Check sheet for the modelled part. Datum: model origin and axes. Units: mm. A direction names the side the tool comes from. Round coordinates to 2 decimals unless told otherwise and drop trailing zeros. Write each loop counter-clockwise with the first axis right and the second up, starting at its lowest first coordinate (ties: lowest second). Pieces come first, ordered by that corner, then holes. Notation, with made-up numbers: (71.5, 24) - (116.5, 24) arc R4 cw to (116.5, 28) - close; hole circle Ø3 at (-5, 74). An arc over 180 degrees is marked (long way). Answer as a JSON object with one key per item and string values. Group by question number.
Item 1: Sectioned sample at C-C on x = 1.25. Record the boundary of the cut face in (y, z), plus the area to 3 significant figures.
Item 2: Sectioned sample at B-B on y = 2.5. Record the boundary of the cut face in (x, z).
Item 3: Sectioned sample at A-A on x = 6.25. Record the boundary of the cut face in (y, z).
Item 4: Gauge pin test, flat ends, axial feed: P1, Ø2.5, axis at y = 0, z = 7, coming from the +X side; P2, Ø1.5, axis at x = 1.5, z = 5, coming from the -Y side; P3, Ø8, axis at y = 6, z = 13.5, coming from the +X side. Record the tip position at first contact, or that the pin passes through.
Item 5: Release check for a two-part mould opening along Y. For faces 1 (the flat face through (5.458, -4.067, 9.86)), 2 (the flat face through (-2.75, 0, 10)), 3 (the flat face through (0.1, 3.4, 0)) record: pulls with the +Y half, pulls with the -Y half, needs draft (parallel to the pull), parting line crosses it, or undercut.
Item 6: Thickness scan on line 1 (X direction, y = 1, z = 13.5); line 2 (Y direction, x = 2.5, z = 10.5); line 3 (X direction, y = 2.5, z = 11.25). Record the ranges inside material, lowest first.
Item 7: Set-up check for faces 4 (the flat face through (-2.69, 6.25, 9.86)), 5 (the flat face through (-6.74, -0.815, 9.86)), 6 (the flat face through (-1.394, -2.37, 9.86)): record each of +Z, -Z, +X, -X, +Y, -Y from which the full face is reachable in a straight line by a thin tool's end or side.
```python
from build123d import *

# Parameters (mm, degrees)
PAD_DEPTH = 20


with BuildPart() as part:
    # Sketch → Pad (new body)
    with BuildSketch(Plane.XY):
        Polygon((-3.75, 6.495191), (-1.607695, 6), (0, 7.5), (1.607695, 6), (3.75, 6.495191), (4.392305, 4.392305), (6.495191, 3.75), (6, 1.607695), (7.5, 0), (6, -1.607695), (6.495191, -3.75), (4.392305, -4.392305), (3.75, -6.495191), (1.607695, -6), (0, -7.5), (-1.607695, -6), (-3.75, -6.495191), (-4.392305, -4.392305), (-6.495191, -3.75), (-6, -1.607695), (-7.5, 0), (-6, 1.607695), (-6.495191, 3.75), (-4.392305, 4.392305), align=None)
        Polygon((2.75, 1.587713), (0, 3.175426), (-2.75, 1.587713), (-2.75, -1.587713), (0, -3.175426), (2.75, -1.587713), align=None, mode=Mode.SUBTRACT)
    extrude(amount=PAD_DEPTH)


solid = part.part
```
Completed:
{
 "1": {"outline": "(-6.33, 0) - (-2.45, 0) - (-2.45, 20) - (-6.33, 20) - close; (2.45, 0) - (6.33, 0) - (6.33, 20) - (2.45, 20) - close", "area": "155 mm²"},
 "2": {"outline": "(-6.21, 0) - (-1.17, 0) - (-1.17, 20) - (-6.21, 20) - close; (1.17, 0) - (6.21, 0) - (6.21, 20) - (1.17, 20) - close"},
 "3": {"outline": "(-3.82, 0) - (-2.69, 0) - (-2.69, 20) - (-3.82, 20) - close; (-1.34, 0) - (1.34, 0) - (1.34, 20) - (-1.34, 20) - close; (2.69, 0) - (3.82, 0) - (3.82, 20) - (2.69, 20) - close"},
 "4": {"P1": "x = 7.5", "P2": "y = -6.8", "P3": "x = 6.5"},
 "5": {"face 1": "pulls with the -Y half", "face 2": "undercut", "face 3": "needs draft"},
 "6": {"line 1": "-6.57 to -2.75, 2.75 to 6.57", "line 2": "-6.21 to -1.73, 1.73 to 6.21", "line 3": "-6.21 to -1.17, 1.17 to 6.21"},
 "7": {"face 4": "+Z, -Z, +Y", "face 5": "+Z, -Z, -X", "face 6": "+Z, -Z"}
}
